Geometry: final body of the model. Coordinates: model frame, mm. Give positions to 0.01 mm unless a question says otherwise; leave off trailing zeros. Order: outer loops, then holes, each group sorted by start corner. A loop starts at its lowest first (then second) coordinate and runs counter-clockwise, first axis right, second up. Notation, with made-up numbers: (37.25, 3) -> (85.25, 3) arc R14 ccw to (85.25, 15) -> close; hole circle Ø7 at (60, -5). An arc over 180 degrees is marked (long way). One line per question, with ' | ' between items.
from build123d import *

# Parameters (mm, degrees)
SKETCH2_R          = 1.73355
CUT_EXTRUDE1_DEPTH = 3.9845
CHAMFER1_SIZE      = 0.1778


with BuildPart() as part:
    # Sketch1 → Revolve1 (revolve)
    with BuildSketch(Plane(origin=(0, 0, 0), x_dir=(1, 0, 0), z_dir=(0, 1, 0))):
        Polygon((0, 0), (3.175, 0), (3.175, 2.032), (2.2225, 2.9845), (0, 2.9845), align=None)
    revolve(axis=Axis((0, 0, 0), (0, 0, 1)))

    # Sketch2 → Cut-Extrude1 (cut, through all)
    with BuildSketch(Plane(origin=(0, 0, -2.9845), x_dir=(-1, 0, 0), z_dir=(0, 0, -1))):
        Circle(SKETCH2_R)
    extrude(amount=-CUT_EXTRUDE1_DEPTH, mode=Mode.SUBTRACT)

    # Chamfer1
    chamfer1_edges = [part.edges().sort_by_distance(p)[0] for p in [
        (-3.175, 0, 0),
    ]]
    chamfer(chamfer1_edges, length=CHAMFER1_SIZE)


solid = part.part
1) Contact query for flat-ended pins moving along their axis: pin 1 Ø1 at (x, z) = (-1, -2) entering from +Y; pin 2 Ø3 at (x, y) = (0, 0) entering from -Z. Output: stop coordinate, or through.
Check result:
pin 1: stops at y = 3.14 | pin 2: passes through
2) Section C-C on z = -1.85. Return loops of the section in (x, y) (3 decimals).
Check result:
outline: circle Ø6.35 at (0, 0); hole circle Ø3.467 at (0, 0)
3) Section D-D on z = -2.35. Return loops of the section in (x, y), plus the area to 3 significant figures.
Check result:
outline: circle Ø5.71 at (0, 0); hole circle Ø3.47 at (0, 0) | area: 16.2 mm^2
4) Pull-direction query (Y, two-part tool) for faces 1 (the cylindrical face through (-0.932, 1.462, -1.513)), 2 (the cylindrical face through (-0.69, -3.1, -1.12)), 3 (the flat face through (0, -2, -2.984)); classes: +Y half, -Y half, draft (parallel to the pull), parting line (faces both ways), or undercut.
Check result:
face 1: undercut | face 2: parting line | face 3: draft
5) Material intervals for probe 1 along Y at (x, z) = (0, -1.85) (3 decimals); probe 2 along Y at (x, z) = (1.5, -0.9); probe 3 along X at (y, z) = (-1.25, -1.9), sorted ascending. Write a range as from..to.
Check result:
probe 1: y = -3.175..-1.734, 1.734..3.175 | probe 2: y = -2.8..-0.87, 0.87..2.8 | probe 3: x = -2.92..-1.2, 1.2..2.92
